CAD build for the part. Positions are in the model's coordinates, mm. Round coordinates to 2 decimals unless told otherwise and drop trailing zeros. Write each loop counter-clockwise with the first axis right and the second up, starting at its lowest first coordinate (ties: lowest second). Pieces come first, ordered by that corner, then holes. Notation, with made-up numbers: (64, 26) - (112, 26) arc R8 cw to (112, 31) - close; hole circle Ø5 at (63, 76). An arc over 180 degrees is marked (long way). Answer in a Markdown table with one row per item.
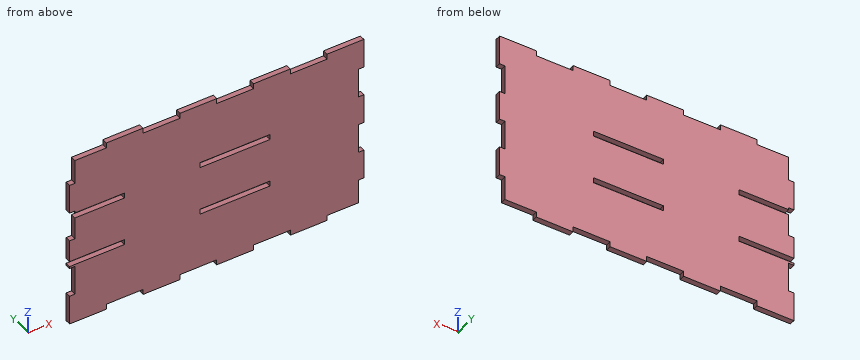
```python
from build123d import *

# Parameters (mm, degrees)
SKETCH1_W           = 59.517928736
SKETCH1_H           = 4.5593
BOSS_EXTRUDE1_DEPTH = 4.5593


with BuildPart() as part:
    # Sketch1 → Boss-Extrude1 (new body)
    with BuildSketch(Plane(origin=(0, 0, 0), x_dir=(1, 0, 0), z_dir=(0, 1, 0))):
        Polygon((-100.66298534, 77.9907), (-131.93673534, 77.9907), (-131.93673534, 52.5907), (-127.37743534, 52.5907), (-127.37743534, 27.1907), (-131.93673534, 27.1907), (-131.93673534, 25.4), (-85.368575998, 25.4), (-85.368575998, 20.8407), (-131.93673534, 20.8407), (-131.93673534, 1.7907), (-127.37743534, 1.7907), (-127.37743534, -17.2593), (-85.368575998, -17.2593), (-85.368575998, -21.8186), (-127.37743534, -21.8186), (-127.37743534, -23.6093), (-131.93673534, -23.6093), (-131.93673534, -49.0093), (-127.37743534, -49.0093), (-127.37743534, -69.85), (-100.66298534, -69.85), (-100.66298534, -74.4093), (-69.38923534, -74.4093), (-69.38923534, -69.85), (-38.11548534, -69.85), (-38.11548534, -74.4093), (-6.84173534, -74.4093), (-6.84173534, -69.85), (24.43201466, -69.85), (24.43201466, -74.4093), (55.70576466, -74.4093), (55.70576466, -69.85), (86.97951466, -69.85), (86.97951466, -74.4093), (118.25326466, -74.4093), (118.25326466, -49.0093), (113.69396466, -49.0093), (113.69396466, -23.6093), (118.25326466, -23.6093), (118.25326466, 1.7907), (113.69396466, 1.7907), (113.69396466, 27.1907), (118.25326466, 27.1907), (118.25326466, 52.5907), (113.69396466, 52.5907), (113.69396466, 73.4314), (86.97951466, 73.4314), (86.97951466, 77.9907), (55.70576466, 77.9907), (55.70576466, 73.4314), (24.43201466, 73.4314), (24.43201466, 77.9907), (-6.84173534, 77.9907), (-6.84173534, 73.4314), (-38.11548534, 73.4314), (-38.11548534, 77.9907), (-69.38923534, 77.9907), (-69.38923534, 73.4314), (-100.66298534, 73.4314), align=None)
        with Locations((8.690322735, -19.53895)):
            Rectangle(SKETCH1_W, SKETCH1_H, mode=Mode.SUBTRACT)
        with Locations((8.690322735, 23.12035)):
            Rectangle(SKETCH1_W, SKETCH1_H, mode=Mode.SUBTRACT)
    extrude(amount=BOSS_EXTRUDE1_DEPTH)


solid = part.part
```
Q1. Saw through at C-C on y = 2.65. Count the separate pieces of the cut face and the enclosed holes in it, then the cut area to 3 significant figures.
Computed:
| item | result |
|---|---|
| separate pieces | 1 |
| enclosed holes | 2 |
| area | 35,400 mm2 |
Q2. Saw through at B-B on z = 1. List the corners of the cut face in (x, y).
Computed:
| item | result |
|---|---|
| outline | (-127.38, 0) - (118.25, 0) - (118.25, 4.56) - (-127.38, 4.56) - close |
Q3. Saw through at A-A on x = -97. List the corners of the cut face in (y, z).
Computed:
| item | result |
|---|---|
| outline | (0, -73.43) - (4.56, -73.43) - (4.56, -25.4) - (0, -25.4) - close; (0, -20.84) - (4.56, -20.84) - (4.56, 17.26) - (0, 17.26) - close; (0, 21.82) - (4.56, 21.82) - (4.56, 74.41) - (0, 74.41) - close |
Q4. Flat gauge pins, fed straight in: pin 1 (2.5 mm diameter, centred on y = 2, z = 19.5, fed in from -X); pin 2 (1.4 mm diameter, centred on x = 115.5, y = 2.5, fed in from -Z); pin 3 (1.4 mm diameter, centred on x = -79.5, y = 2, fed in from -Z). Where does each tip first touch, or does it go through?
Computed:
| item | result |
|---|---|
| pin 1 | stops at x = -85.37 |
| pin 2 | stops at z = -52.59 |
| pin 3 | stops at z = -73.43 |
Q5. Drill centre lines: line 1 (Z direction, x = 12, y = 2.7); line 2 (Z direction, x = -13, y = 1.1); line 3 (X direction, y = 2.2, z = -42.5). Where is each one in solid material? Low to high.
Computed:
| item | result |
|---|---|
| line 1 | z = -77.99 to -25.4, -20.84 to 17.26, 21.82 to 69.85 |
| line 2 | z = -73.43 to -25.4, -20.84 to 17.26, 21.82 to 74.41 |
| line 3 | x = -127.38 to 118.25 |
Q6. Saw through at D-D on x = 79.5. List the corners of the cut face in (y, z), then the cut area to 3 significant figures.
Computed:
| item | result |
|---|---|
| outline | (0, -77.99) - (4.56, -77.99) - (4.56, 69.85) - (0, 69.85) - close |
| area | 674 mm2 |
